The listing builds one solid part. Answer for the finished solid, in the listing's coordinates (mm). Face numbers are marked on the shaded views. A direction names the side the tool comes from. Coordinates: 2 decimals unless noted, no trailing zeros. Order: outer loops, then holes, each group sorted by start corner. A loop starts at its lowest first (then second) coordinate and runs counter-clockwise, first axis right, second up. Notation, with made-up numbers: M -27.5,61 L -11.5,61 A9 cw -11.5,67 Z; hole C -31,-15.5 d3. An arc over 180 degrees is marked long. One line per item, written item: value. Start each with the question number.
Q1. The part is cut by section A-A on z = 10.5. Give the vertices of the cut face in (x, y), then the cut area to 3 significant figures.
Q2. Determine the mould class of the marked faces 3, 4 and 5 for opening direction Z: pulls with the +Z half, pulls with the -Z half, needs draft (parallel to the pull), parting line crosses it, or undercut.
Q3. The part is cut by section C-C on x = -31.5. Give the vertices of the cut face in (y, z).
Q4. For the marked faces 1 and 2, determine the directions among +Z, -Z, +X, -X, +Y, -Y from which every point of the face is accessible in a straight line to the end or side of a thin tool.
Q5. The part is cut by section B-B on y = 1.25. Give the vertices of the cut face in (x, z).
Q6. Straight lines are drawn through the part: line 1 along X through (y, z) = (1.6, -7); line 2 along Z through (x, y) = (-34, 2.85); line 3 along Z through (x, y) = (-9.5, 1.05). For each, find the intervals that lie inside material, in ascending order. Write a range as [from, to].
```python
from build123d import *

# Parameters (mm, degrees)
EXTRUDE_3_DEPTH     = 5
SKETCH_7_R          = 1.5
CUT_EXTRUDE_1_DEPTH = 62.435637135
SKETCH_8_W          = 45
SKETCH_8_H          = 35
CUT_EXTRUDE_2_DEPTH = 62.435637135


with BuildPart() as part:
    # 草图1 → 凸台-拉伸3 (new body)
    with BuildSketch(Plane(origin=(0, 0, 0), x_dir=(1, 0, 0), z_dir=(0, 1, 0))):
        with BuildLine():
            Line((-55.213994356, 19.544380587), (-10.213994356, 19.544380587))
            ThreePointArc((-10.213994356, 19.544380587), (-8.446227403, 18.81214754), (-7.713994356, 17.044380587))
            Line((-7.713994356, 17.044380587), (-7.713994356, -17.955619413))
            ThreePointArc((-7.713994356, -17.955619413), (-8.446227403, -19.723386366), (-10.213994356, -20.455619413))
            Line((-10.213994356, -20.455619413), (-55.213994356, -20.455619413))
            ThreePointArc((-55.213994356, -20.455619413), (-56.981761309, -19.723386366), (-57.713994356, -17.955619413))
            Line((-57.713994356, -17.955619413), (-57.713994356, 17.044380587))
            ThreePointArc((-57.713994356, 17.044380587), (-56.981761309, 18.81214754), (-55.213994356, 19.544380587))
        make_face()
    extrude(amount=EXTRUDE_3_DEPTH)

    # 草图7 → 切除-拉伸1 (cut, through all)
    with BuildSketch(Plane(origin=(0, 5, 0), x_dir=(1, 0, 0), z_dir=(0, 1, 0))):
        with Locations(Location((-55.213994356, 17.044380587, 0), (0, 0, 270))):
            Circle(SKETCH_7_R)
        with Locations(Location((-10.213994356, 17.044380587, 0), (0, 0, 270))):
            Circle(SKETCH_7_R)
        with Locations(Location((-55.213994356, -17.955619413, 0), (0, 0, 270))):
            Circle(SKETCH_7_R)
        with Locations(Location((-10.213994356, -17.955619413, 0), (0, 0, 270))):
            Circle(SKETCH_7_R)
    extrude(amount=-CUT_EXTRUDE_1_DEPTH, mode=Mode.SUBTRACT)

    # 草图8 → 切除-拉伸2 (cut, through all)
    with BuildSketch(Plane(origin=(0, 5, 0), x_dir=(1, 0, 0), z_dir=(0, 1, 0))):
        with Locations((-32.713994356, -0.455619413)):
            Rectangle(SKETCH_8_W, SKETCH_8_H)
    extrude(amount=-CUT_EXTRUDE_2_DEPTH, mode=Mode.SUBTRACT)


solid = part.part
```
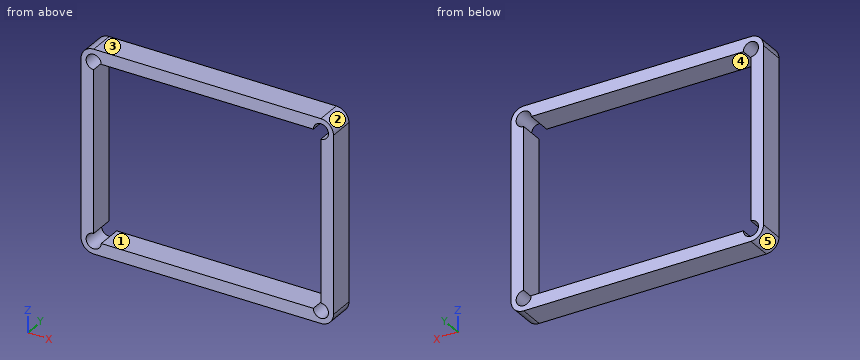
Output:
1. outline: M -57.71,0 L -55.21,0 L -55.21,5 L -57.71,5 Z; M -10.21,0 L -7.71,0 L -7.71,5 L -10.21,5 Z
1. area: 25.0 mm^2
2. face 3: pulls with the +Z half
2. face 4: undercut
2. face 5: pulls with the -Z half
3. outline: M 0,-19.54 L 5,-19.54 L 5,-17.04 L 0,-17.04 Z; M 0,17.96 L 5,17.96 L 5,20.46 L 0,20.46 Z
4. face 1: +Y, -Y
4. face 2: +Z, +X, +Y, -Y
5. outline: M -57.71,-17.04 A2.5 ccw -55.21,-19.54 L -10.21,-19.54 A2.5 ccw -7.71,-17.04 L -7.71,17.96 A2.5 ccw -10.21,20.46 L -55.21,20.46 A2.5 ccw -57.71,17.96 Z; hole M -55.21,-15.54 A1.5 ccw long -53.71,-17.04 L -11.71,-17.04 A1.5 ccw long -10.21,-15.54 L -10.21,16.46 A1.5 ccw long -11.71,17.96 L -53.71,17.96 A1.5 ccw long -55.21,16.46 Z
6. line 1: x = [-57.71, -55.21], [-10.21, -7.71]
6. line 2: z = [-19.54, -17.04], [17.96, 20.46]
6. line 3: z = [-19.44, -18.36], [-15.73, 16.64], [19.27, 20.35]
